from build123d import *

# Parameters (mm, degrees)
BOSS_EXTRUDE1_DEPTH              = 3.175
SKETCH4_R                        = 15.875
CUT_EXTRUDE1_DEPTH               = 4.175
SKETCH10_R                       = 2.0955
CUT_EXTRUDE5_DEPTH               = 4.175
CUT_EXTRUDE6_DEPTH               = 3.175
SKETCH12_R                       = 2.0193
CUT_EXTRUDE7_DEPTH               = 3.175
F_25_64_0_39063_DIAMETER_HOLE1_D = 9.922002


with BuildPart() as part:
    # Sketch1 → Boss-Extrude1 (new body)
    with BuildSketch(Plane.XY):
        with BuildLine():
            Line((-127.585439757, -38.931312956), (20.895912371, -38.931312956))
            ThreePointArc((20.895912371, -38.931312956), (63.319116371, -25.555328115), (90.398020935, 9.734587382))
            Line((90.398020935, 9.734587382), (99.264008145, 34.093687044))
            Line((99.264008145, 34.093687044), (69.069421488, 8.757420515))
            ThreePointArc((69.069421488, 8.757420515), (58.622007829, 5.045238426), (48.293203475, 9.075691085))
            Line((48.293203475, 9.075691085), (-39.53568268, 87.480536572))
            Line((-39.53568268, 87.480536572), (-3.340712695, 109.466412576))
            ThreePointArc((-3.340712695, 109.466412576), (-35.575547408, 122.196999074), (-69.251886775, 114.008191568))
            ThreePointArc((-69.251886775, 114.008191568), (-93.222829654, 95.410668155), (-112.371322471, 71.877517018))
            ThreePointArc((-112.371322471, 71.877517018), (-128.087342247, 59.948856215), (-147.787037557, 61.048051754))
            Line((-147.787037557, 61.048051754), (-177.372260989, 73.844569494))
            Line((-177.372260989, 73.844569494), (-276.451380272, 116.699331448))
            ThreePointArc((-276.451380272, 116.699331448), (-297.183919754, 38.884009246), (-276.451380272, -38.931312956))
            Line((-276.451380272, -38.931312956), (-127.585439757, -38.931312956))
        make_face()
    extrude(amount=BOSS_EXTRUDE1_DEPTH)

    # Sketch4 → Cut-Extrude1 (cut, through all)
    with BuildSketch(Plane.XY):
        with Locations((-19.051033526, -2.418812956)):
            Circle(SKETCH4_R)
    extrude(amount=CUT_EXTRUDE1_DEPTH, mode=Mode.SUBTRACT)

    # Sketch10 → Cut-Extrude5 (cut, through all)
    with BuildSketch(Plane.XY.offset(3.175)):
        with Locations((-97.11436, -26.231312956)):
            Circle(SKETCH10_R)
        with Locations((-71.71436, -26.231312956)):
            Circle(SKETCH10_R)
        with Locations((-122.51436, -0.831312956)):
            Circle(SKETCH10_R)
        with Locations((-97.11436, -0.831312956)):
            Circle(SKETCH10_R)
    extrude(amount=-CUT_EXTRUDE5_DEPTH, mode=Mode.SUBTRACT)

    # Sketch11 → Cut-Extrude6 (cut)
    with BuildSketch(Plane.XY.offset(3.175)):
        with BuildLine():
            Line((-165.387218926, -25.088312956), (-146.337218926, -25.088312956))
            ThreePointArc((-146.337218926, -25.088312956), (-143.035218926, -21.786312956), (-146.337218926, -18.484312956))
            Line((-146.337218926, -18.484312956), (-165.387218926, -18.484312956))
            ThreePointArc((-165.387218926, -18.484312956), (-168.689218926, -21.786312956), (-165.387218926, -25.088312956))
        make_face()
        with BuildLine():
            Line((-165.387218926, 29.140687044), (-146.337218926, 29.140687044))
            ThreePointArc((-146.337218926, 29.140687044), (-143.035218926, 25.838687044), (-146.337218926, 22.536687044))
            Line((-146.337218926, 22.536687044), (-165.387218926, 22.536687044))
            ThreePointArc((-165.387218926, 22.536687044), (-168.689218926, 25.838687044), (-165.387218926, 29.140687044))
        make_face()
    extrude(amount=-CUT_EXTRUDE6_DEPTH, mode=Mode.SUBTRACT)

    # Sketch12 → Cut-Extrude7 (cut)
    with BuildSketch(Plane.XY.offset(3.175)):
        with Locations((26.111583591, -6.330574271)):
            Circle(SKETCH12_R)
        with Locations((-38.190866701, 8.693687044)):
            Circle(SKETCH12_R)
        with Locations((-47.354412394, -29.406312956)):
            Circle(SKETCH12_R)
        with Locations((26.111583591, -29.406312956)):
            Circle(SKETCH12_R)
    extrude(amount=-CUT_EXTRUDE7_DEPTH, mode=Mode.SUBTRACT)

    # 25/64 (0.39063) Diameter Hole1 (through all)
    with Locations(Plane.XY.offset(3.175)):
        with Locations((-28.740712695, 108.89709501), (-93.867251666, 69.337343725)):
            Hole(F_25_64_0_39063_DIAMETER_HOLE1_D / 2)


solid = part.part
Here's how the part is built. I have some questions about the finished solid (model axes, mm). A direction names the side the tool comes from. Give positions to 0.01 mm unless a question says otherwise; leave off trailing zeros. Loops run counter-clockwise (first coordinate to the right, second up) from the corner with the lowest first, then second, coordinate; pieces in that order, holes last. Notation, with made-up numbers: (-10, 13.25) -> (31, 13.25) arc R11 ccw to (31, 23.25) -> close; hole circle Ø2 at (27.25, -34). An arc over 180 degrees is marked (long way). One line per item, written item: value.
Q1. Suppose I cut it at B-B on z = 2.6. State how many separate pieces and enclosed holes the cut face has, then the cut area to 3 significant figures.
Answers follow:
separate pieces: 1
enclosed holes: 13
area: 41,000 mm^2
Q2. Suppose I cut it at C-C on x = -156. Please give me the cut outline in (y, z) (3 decimals), then the cut area to 3 significant figures.
Answers follow:
outline: (-38.931, 0) -> (-25.088, 0) -> (-25.088, 3.175) -> (-38.931, 3.175) -> close; (-18.484, 0) -> (22.537, 0) -> (22.537, 3.175) -> (-18.484, 3.175) -> close; (29.141, 0) -> (64.6, 0) -> (64.6, 3.175) -> (29.141, 3.175) -> close
area: 287 mm^2
Q3. Suppose I cut it at A-A on y = 96. Please give me the cut outline in (x, z) (3 decimals), then the cut area to 3 significant figures.
Answers follow:
outline: (-286.382, 0) -> (-228.595, 0) -> (-228.595, 3.175) -> (-286.382, 3.175) -> close; (-92.616, 0) -> (-25.51, 0) -> (-25.51, 3.175) -> (-92.616, 3.175) -> close
area: 397 mm^2
Q4. Suppose I cut it at D-D on x = 56. Please give me the cut outline in (y, z) (3 decimals).
Answers follow:
outline: (-30.07, 0) -> (5.304, 0) -> (5.304, 3.175) -> (-30.07, 3.175) -> close
Q5. We'd pull the mould along Y, two halves only. Please class faces 6 (the face through (84.378, 21.603, 1.565)), 7 (the face through (-30.75, 8.31, 1.57)), 8 (the face through (-297.18, 40.02, 1.57)): pulls with the +Y half, pulls with the -Y half, needs draft (parallel to the pull), parting line crosses it, or undercut.
Answers follow:
face 6: pulls with the +Y half
face 7: undercut
face 8: parting line crosses it
Q6. On a 3-axis mill with a long thin cutter (end or side, diameter ignored), from which of +Z, -Z, +X, -X, +Y, -Y can I reach the whole of each face in a straight line? I mean faces 1 (the face through (-21.69, 98.32, 1.57)), 2 (the face through (-146, 43, 0)), 3 (the face through (-146, 43, 3.175)), 4 (the face through (4.99, 47.73, 1.57)), 5 (the face through (-92.918, 95.708, 1.565)). Say none if no direction works.
Answers follow:
face 1: +Z, -Z, +X
face 2: -Z, +X, -X, +Y, -Y
face 3: +Z, +X, -X, +Y, -Y
face 4: +Z, -Z
face 5: +Z, -Z, +Y
Q7. If I drill on line 1 along X through (y, z) = (-26.5, 0.6); line 2 along Y through (x, z) = (-13, 1.3); line 3 along Y through (x, z) = (-5.5, 1.65), over which ranges is the centre line in solid material (lowest first)?
Answers follow:
line 1: -282.86 to -99.19, -95.04 to -73.79, -69.64 to 61.94
line 2: -38.93 to -17.1, 12.26 to 63.79, 103.6 to 115.83
line 3: -38.93 to -10.69, 5.85 to 57.1, 108.15 to 111.14
Q8. I'm going to push flat-ended pins straight in: pin 1 Ø1 at (x, z) = (-152, 2) entering from +Y; pin 2 Ø4.5 at (x, y) = (-47.35, -29.41) entering from +Z (3 decimals); pin 3 Ø1 at (y, z) = (27, 1.5) entering from -X; pin 4 Ø1.6 at (x, z) = (-151, 1.5) entering from +Y. Where does each tip first touch, or does it pass through?
Answers follow:
pin 1: y = 63.09
pin 2: z = 3.175
pin 3: x = -296.77
pin 4: y = 62.78
